Build history of the part. All positions in model axes, mm. A direction names the side the tool comes from. Round coordinates to 2 decimals unless told otherwise and drop trailing zeros. Loops run counter-clockwise (first coordinate to the right, second up) from the corner with the lowest first, then second, coordinate; pieces in that order, holes last. Notation, with made-up numbers: (31.5, -6) -> (54.5, -6) arc R11 ccw to (54.5, 13) -> close; hole circle Ø10 at (38.25, -10). An arc over 180 degrees is marked (long way). Put each result on its own line as item: value. Start each with the question number.
```python
from build123d import *

# Parameters (mm, degrees)
SKETCH1_R           = 4
BOSS_EXTRUDE1_DEPTH = 5
BOSS_EXTRUDE2_DEPTH = 7
SKETCH3_R           = 4
BOSS_EXTRUDE3_DEPTH = 5
BOSS_EXTRUDE4_START = -13.5
BOSS_EXTRUDE4_DEPTH = 10
FILLET1_R           = 10
SKETCH7_W           = 20
SKETCH7_H           = 20
BOSS_EXTRUDE6_DEPTH = 20
SKETCH8_R           = 7.5
CUT_EXTRUDE2_DEPTH  = 20


with BuildPart() as part:
    # Sketch1 → Boss-Extrude1 (new body)
    with BuildSketch(Plane.XY):
        with BuildLine():
            Line((-50, 0), (-10, 0))
            ThreePointArc((-10, 0), (0, 10), (10, 0))
            Line((10, 0), (50, 0))
            ThreePointArc((50, 0), (0, -50), (-50, 0))
        make_face()
        Circle(SKETCH1_R, mode=Mode.SUBTRACT)
    extrude(amount=BOSS_EXTRUDE1_DEPTH)

    # Sketch2 → Boss-Extrude2 (add)
    with BuildSketch(Plane.XY.offset(5)):
        with BuildLine():
            Line((-50, 0), (-40, 0))
            ThreePointArc((-40, 0), (0, -40), (40, 0))
            Line((40, 0), (50, 0))
            ThreePointArc((50, 0), (0, -50), (-50, 0))
        make_face()
    extrude(amount=BOSS_EXTRUDE2_DEPTH)

    # Sketch3 → Boss-Extrude3 (add)
    with BuildSketch(Plane.XY.offset(12)):
        with BuildLine():
            Line((-50, 0), (-10, 0))
            ThreePointArc((-10, 0), (0, 10), (10, 0))
            Line((10, 0), (50, 0))
            ThreePointArc((50, 0), (0, -50), (-50, 0))
        make_face()
        Circle(SKETCH3_R, mode=Mode.SUBTRACT)
    extrude(amount=BOSS_EXTRUDE3_DEPTH)

    # Sketch4 → Boss-Extrude4 (add)
    with BuildSketch(Plane.XY.offset(17).offset(BOSS_EXTRUDE4_START)):
        with BuildLine():
            Line((-10, -95), (10, -95))
            Line((10, -95), (10, -90))
            Line((10, -90), (48.299537742, -90))
            Line((48.299537742, -90), (48.299537742, -12.928830338))
            ThreePointArc((48.299537742, -12.928830338), (44.35247464, -23.08371706), (38.299537742, -32.142579373))
            Line((38.299537742, -32.142579373), (38.299537742, -80))
            Line((38.299537742, -80), (10, -80))
            Line((10, -80), (10, -75))
            Line((10, -75), (-10, -75))
            Line((-10, -75), (-10, -80))
            Line((-10, -80), (-38.299537742, -80))
            Line((-38.299537742, -80), (-38.299537742, -32.142579373))
            ThreePointArc((-38.299537742, -32.142579373), (-44.35247464, -23.08371706), (-48.299537742, -12.928830338))
            Line((-48.299537742, -12.928830338), (-48.299537742, -90))
            Line((-48.299537742, -90), (-10, -90))
            Line((-10, -90), (-10, -95))
        make_face()
    extrude(amount=BOSS_EXTRUDE4_DEPTH)

    # Fillet1
    fillet1_edges = [part.edges().sort_by_distance(p)[0] for p in [
        (48.299537742, -90, 8.5),
        (-48.299537742, -90, 8.5),
    ]]
    fillet(fillet1_edges, radius=FILLET1_R)

    # Sketch7 → Boss-Extrude6 (add)
    with BuildSketch(Plane.XZ.offset(95)):
        with Locations((0, 8.5)):
            Rectangle(SKETCH7_W, SKETCH7_H)
    extrude(amount=-BOSS_EXTRUDE6_DEPTH)

    # Sketch8 → Cut-Extrude2 (cut)
    with BuildSketch(Plane.XZ.offset(95)):
        with Locations(Location((0, 8.5, 0), (0, 0, 270))):
            Circle(SKETCH8_R)
    extrude(amount=-CUT_EXTRUDE2_DEPTH, mode=Mode.SUBTRACT)


solid = part.part
```
Item 1: Cut at C-C on y = -81.5. Write the cut outline in (x, z).
Item 2: Pull direction Z, two halves, no side cores. Call faces 1 (the face through (-0.88, -39.99, 8.45)), 2 (the face through (-39, -63, 3.5)), 3 (the face through (24, -90, 8)), 4 (the face through (1, -15, 12)): +Z half, -Z half, draft (parallel to the pull), parting line (faces both ways), or undercut.
Item 3: Cut at B-B on x = 0. Write the cut outline in (y, z), then the cut area to 3 significant figures.
Item 4: Cut at A-A on y = -57. Write the cut outline in (x, z), then the cut area to 3 significant figures.
Item 5: Drop flat-ended pins along their axis: pin 1 (10.5 mm diameter, centred on x = 0, y = 0, fed in from +Z); pin 2 (3 mm diameter, centred on y = -66, z = 7, fed in from +X); pin 3 (15 mm diameter, centred on x = -4, y = -13.5, fed in from -Z). Give the stop position or say it passes through.
Item 6: Wall check: line 1 (Z direction, x = 31.5, y = -10); line 2 (Z direction, x = 30, y = -38); line 3 (Y direction, x = 0, z = 15.3). Give the ranges that are in metal, low to high. Write a range as from..to.
Item 7: Cut at D-D on x = -35.5. Write the cut outline in (y, z), then the cut area to 3 significant figures.
Item 8: 3-axis set-ups, long thin cutter, end or side, ignore diameter. For faces 5 (the face through (-30.3, 0, 4.6)), 6 (the face through (39, -66, 13.5)), 7 (the face through (39, -66, 3.5)), 8 (the face through (48.3, -47, 8)): which of +Z, -Z, +X, -X, +Y, -Y reach the whole face in a straight line?
Ans:
1. outline: (-48.19, 3.5) -> (-10, 3.5) -> (-10, -1.5) -> (10, -1.5) -> (10, 3.5) -> (48.19, 3.5) -> (48.19, 13.5) -> (10, 13.5) -> (10, 18.5) -> (-10, 18.5) -> (-10, 13.5) -> (-48.19, 13.5) -> close; hole circle Ø15 at (0, 8.5)
2. face 1: undercut
2. face 2: -Z half
2. face 3: draft
2. face 4: undercut
3. outline: (-95, -1.5) -> (-75, -1.5) -> (-75, 1) -> (-95, 1) -> close; (-95, 16) -> (-75, 16) -> (-75, 18.5) -> (-95, 18.5) -> close; (-50, 0) -> (-4, 0) -> (-4, 5) -> (-40, 5) -> (-40, 12) -> (-4, 12) -> (-4, 17) -> (-50, 17) -> close; (4, 0) -> (10, 0) -> (10, 5) -> (4, 5) -> close; (4, 12) -> (10, 12) -> (10, 17) -> (4, 17) -> close
3. area: 690 mm2
4. outline: (-48.3, 3.5) -> (-38.3, 3.5) -> (-38.3, 13.5) -> (-48.3, 13.5) -> close; (38.3, 3.5) -> (48.3, 3.5) -> (48.3, 13.5) -> (38.3, 13.5) -> close
4. area: 200 mm2
5. pin 1: stops at z = 17
5. pin 2: stops at x = 48.3
5. pin 3: stops at z = 0
6. line 1: z = 0..5, 12..17
6. line 2: z = 0..17
6. line 3: y = -50..-4, 4..10
7. outline: (-90, 3.5) -> (-80, 3.5) -> (-80, 13.5) -> (-90, 13.5) -> close; (-35.21, 0) -> (0, 0) -> (0, 5) -> (-18.43, 5) -> (-18.43, 12) -> (0, 12) -> (0, 17) -> (-35.21, 17) -> close
7. area: 570 mm2
8. face 5: +Z, -Z, -X, +Y
8. face 6: +Z, +X, -Y
8. face 7: -Z, +X, -Y
8. face 8: +Z, -Z, +X, -Y
